Check sheet for the drawn part. Datum: minimum x, y, z corner. Units: mm. A direction names the side the tool comes from. Give positions to 0.01 mm unless a question says otherwise; leave off trailing zeros. Write each loop counter-clockwise with the first axis right and the second up, starting at its lowest first coordinate (ties: lowest second). Pieces come first, ordered by that corner, then holes.
(1) Cross-section at A-A (y = 9.5). Record the boundary of the cut face in (x, z), and give its area (3 significant figures).
(2) Thickness scan on line 1 along X through (y, z) = (13, 8.5); line 2 along Z through (x, y) = (11, 35); line 3 along Y through (x, z) = (22, 9.75). Record the ranges inside material, lowest first.
(3) Tool access check on the marked faces 1 and 2. Record the directions out of +Z, -Z, +X, -X, +Y, -Y that give a thin tool (end or side, any length) a straight path to the whole face; none if there is none.
(4) Cross-section at D-D (y = 17). Record the boundary of the cut face in (x, z), and give its area (3 significant figures).
(5) Depth check by flat-ended pin: P1, Ø1.5, axis at x = 53, z = 12, coming from the +Y side; P2, Ø20.5, axis at x = 45.5, y = 35.5, coming from the +Z side; P3, Ø7.5, axis at x = 28.5, y = 36, coming from the -Z side. Enter the tip coordinate at first touch or a pass-through.
(6) Mould release check, pull along X, two halves, no side actions. Record for the marked faces 3, 4 and 5: +X half, -X half, draft (parallel to the pull), parting line (faces both ways), or undercut.
(7) Cross-section at B-B (z = 16). Record the boundary of the cut face in (x, y), and give its area (3 significant figures).
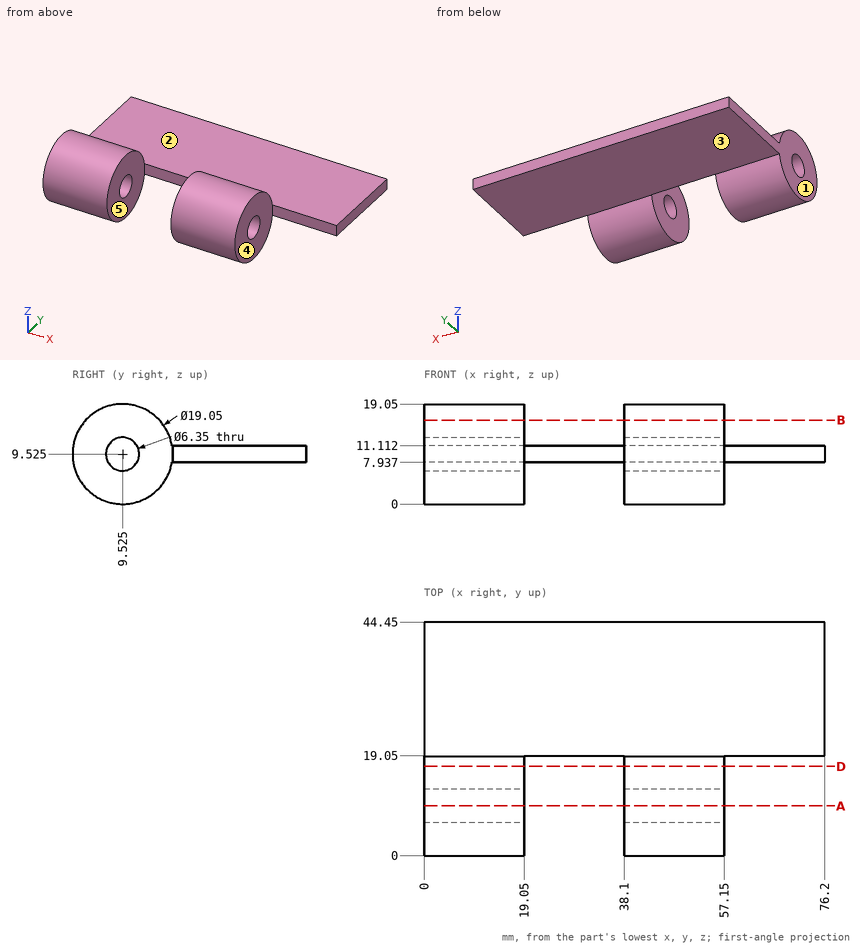
Reply:
1. outline: (0, 0) - (19.05, 0) - (19.05, 6.35) - (0, 6.35) - close; (0, 12.7) - (19.05, 12.7) - (19.05, 19.05) - (0, 19.05) - close; (38.1, 0) - (57.15, 0) - (57.15, 6.35) - (38.1, 6.35) - close; (38.1, 12.7) - (57.15, 12.7) - (57.15, 19.05) - (38.1, 19.05) - close
1. area: 484 mm2
2. line 1: x = 0 to 19.05, 38.1 to 57.15
2. line 2: z = 7.94 to 11.11
2. line 3: y = 19.05 to 44.45
3. face 1: +Z, -Z, -X, +Y, -Y
3. face 2: +Z, +X, -X, +Y
4. outline: (0, 3.62) - (19.05, 3.62) - (19.05, 15.43) - (0, 15.43) - close; (38.1, 3.62) - (57.15, 3.62) - (57.15, 15.43) - (38.1, 15.43) - close
4. area: 450 mm2
5. P1: stops at y = 18.89
5. P2: stops at z = 11.11
5. P3: stops at z = 7.94
6. face 3: draft
6. face 4: +X half
6. face 5: undercut
7. outline: (0, 2.54) - (19.05, 2.54) - (19.05, 16.51) - (0, 16.51) - close; (38.1, 2.54) - (57.15, 2.54) - (57.15, 16.51) - (38.1, 16.51) - close
7. area: 532 mm2
